from build123d import *

# Parameters (mm, degrees)
SKETCH1_4_R         = 20
SKETCH1_4_R_2       = 15
SKETCH1_4_R_3       = 40
SKETCH1_4_R_4       = 32
SKETCH1_4_R_5       = 21
SKETCH1_4_R_6       = 16
BOSS_EXTRUDE2_DEPTH = 17.5
SKETCH1_5_R         = 15
BOSS_EXTRUDE3_DEPTH = 7.5


with BuildPart() as part:
    # Sketch1_4 → Boss-Extrude2 (new, symmetric)
    # profile 1 of 10: a face of its own
    with BuildSketch(Plane.XY):
        with Locations((-70, 0)):
            Circle(SKETCH1_4_R)
        with Locations((-70, 0)):
            Circle(SKETCH1_4_R_2, mode=Mode.SUBTRACT)
    # profile 2 of 10: a face of its own
    with BuildSketch(Plane.XY):
        with Locations((70, 0)):
            Circle(SKETCH1_4_R)
        with Locations((70, 0)):
            Circle(SKETCH1_4_R_2, mode=Mode.SUBTRACT)
    # profile 3 of 10: a face of its own
    with BuildSketch(Plane.XY):
        Circle(SKETCH1_4_R_3)
        Circle(SKETCH1_4_R_4, mode=Mode.SUBTRACT)
    # profile 4 of 10: a face of its own
    with BuildSketch(Plane.XY):
        with BuildLine():
            ThreePointArc((3, 31.859064644), (0, 32), (-3, 31.859064644))
            Line((-3, 31.859064644), (-3, 20.784609691))
            ThreePointArc((-3, 20.784609691), (0, 21), (3, 20.784609691))
            Line((3, 20.784609691), (3, 31.859064644))
        make_face()
    # profile 5 of 10: a face of its own
    with BuildSketch(Plane.XY):
        with BuildLine():
            ThreePointArc((29.090759323, 13.331456111), (27.712812921, 16), (26.090759323, 18.527608533))
            Line((26.090759323, 18.527608533), (16.5, 12.990381057))
            ThreePointArc((16.5, 12.990381057), (18.186533479, 10.5), (19.5, 7.794228634))
            Line((19.5, 7.794228634), (29.090759323, 13.331456111))
        make_face()
    # profile 6 of 10: a face of its own
    with BuildSketch(Plane.XY):
        with BuildLine():
            Line((16.5, -12.990381057), (26.090759323, -18.527608533))
            ThreePointArc((26.090759323, -18.527608533), (27.712812921, -16), (29.090759323, -13.331456111))
            Line((29.090759323, -13.331456111), (19.5, -7.794228634))
            ThreePointArc((19.5, -7.794228634), (18.186533479, -10.5), (16.5, -12.990381057))
        make_face()
    # profile 7 of 10: a face of its own
    with BuildSketch(Plane.XY):
        with BuildLine():
            Line((-3, -20.784609691), (-3, -31.859064644))
            ThreePointArc((-3, -31.859064644), (0, -32), (3, -31.859064644))
            Line((3, -31.859064644), (3, -20.784609691))
            ThreePointArc((3, -20.784609691), (0, -21), (-3, -20.784609691))
        make_face()
    # profile 8 of 10: a face of its own
    with BuildSketch(Plane.XY):
        with BuildLine():
            Line((-19.5, -7.794228634), (-29.090759323, -13.331456111))
            ThreePointArc((-29.090759323, -13.331456111), (-27.712812921, -16), (-26.090759323, -18.527608533))
            Line((-26.090759323, -18.527608533), (-16.5, -12.990381057))
            ThreePointArc((-16.5, -12.990381057), (-18.186533479, -10.5), (-19.5, -7.794228634))
        make_face()
    # profile 9 of 10: a face of its own
    with BuildSketch(Plane.XY):
        with BuildLine():
            ThreePointArc((-26.090759323, 18.527608533), (-27.712812921, 16), (-29.090759323, 13.331456111))
            Line((-29.090759323, 13.331456111), (-19.5, 7.794228634))
            ThreePointArc((-19.5, 7.794228634), (-18.186533479, 10.5), (-16.5, 12.990381057))
            Line((-16.5, 12.990381057), (-26.090759323, 18.527608533))
        make_face()
    # profile 10 of 10: a face of its own
    with BuildSketch(Plane.XY):
        Circle(SKETCH1_4_R_5)
        Circle(SKETCH1_4_R_6, mode=Mode.SUBTRACT)
    extrude(amount=BOSS_EXTRUDE2_DEPTH, both=True)

    # Sketch1_5 → Boss-Extrude3 (add, symmetric)
    # profile 1 of 2: a face of its own
    with BuildSketch(Plane.XY):
        with BuildLine():
            ThreePointArc((-29.089532552, -61.937098635), (-20.55564481, -45.574895377), (-3, -39.88734135))
            ThreePointArc((-3, -39.88734135), (-40, 0), (-3, 39.88734135))
            ThreePointArc((-3, 39.88734135), (-20.55564481, 45.574895377), (-29.089532552, 61.937098635))
            ThreePointArc((-29.089532552, 61.937098635), (-47.761832891, 80.880388119), (-70.02485881, 66.324952937))
            Line((-70.02485881, 66.324952937), (-89.071294105, 6.023764702))
            ThreePointArc((-89.071294105, 6.023764702), (-66.95253237, 19.766460003), (-50, 0))
            ThreePointArc((-50, 0), (-66.95253237, -19.766460003), (-89.071294105, -6.023764702))
            Line((-89.071294105, -6.023764702), (-70.02485881, -66.324952937))
            ThreePointArc((-70.02485881, -66.324952937), (-47.761832891, -80.880388119), (-29.089532552, -61.937098635))
        make_face()
        with Locations((-50, -60)):
            Circle(SKETCH1_5_R, mode=Mode.SUBTRACT)
        with Locations((-50, 60)):
            Circle(SKETCH1_5_R, mode=Mode.SUBTRACT)
    # profile 2 of 2: a face of its own
    with BuildSketch(Plane.XY):
        with BuildLine():
            Line((70.02485881, -66.324952937), (89.071294105, -6.023764702))
            ThreePointArc((89.071294105, -6.023764702), (50, 0), (89.071294105, 6.023764702))
            Line((89.071294105, 6.023764702), (70.02485881, 66.324952937))
            ThreePointArc((70.02485881, 66.324952937), (47.761832891, 80.880388119), (29.089532552, 61.937098635))
            ThreePointArc((29.089532552, 61.937098635), (20.55564481, 45.574895377), (3, 39.88734135))
            ThreePointArc((3, 39.88734135), (29.325756597, 27.202941017), (40, 0))
            ThreePointArc((40, 0), (29.325756597, -27.202941017), (3, -39.88734135))
            ThreePointArc((3, -39.88734135), (20.55564481, -45.574895377), (29.089532552, -61.937098635))
            ThreePointArc((29.089532552, -61.937098635), (47.761832891, -80.880388119), (70.02485881, -66.324952937))
        make_face()
        with Locations((50, -60)):
            Circle(SKETCH1_5_R, mode=Mode.SUBTRACT)
        with Locations((50, 60)):
            Circle(SKETCH1_5_R, mode=Mode.SUBTRACT)
    extrude(amount=BOSS_EXTRUDE3_DEPTH, both=True)


solid = part.part
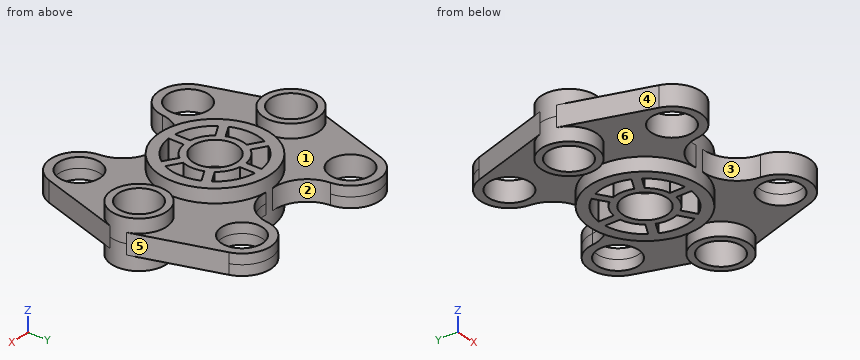
Geometry check sheet. Reference: the model listing, model coordinates, mm. Face numbers are marked on the shaded views. A direction names the side the tool comes from. Give positions to 0.01 mm unless a question says otherwise; leave off trailing zeros. Write each loop counter-clockwise with the first axis right and the second up, starting at its lowest first coordinate (ties: lowest second). Pieces come first, ordered by that corner, then holes.
1) Cross-section at D-D (x = -46). Record the boundary of the cut face in (y, z).
Values follow:
outline: (-80.62, -7.5) - (-74.46, -7.5) - (-74.46, 7.5) - (-80.62, 7.5) - close; (-45.54, -7.5) - (45.54, -7.5) - (45.54, 7.5) - (-45.54, 7.5) - close; (74.46, -7.5) - (80.62, -7.5) - (80.62, 7.5) - (74.46, 7.5) - close
2) Thickness scan on line 1 (Y direction, x = -54.5, z = -2); line 2 (Y direction, x = 39, z = 6.5); line 3 (Y direction, x = -14, z = 13). Record the ranges inside material, lowest first.
Values follow:
line 1: y = -80.51 to -74.31, -45.69 to 45.69, 74.31 to 80.51
line 2: y = -77.89 to -70.2, -49.8 to 49.8, 70.2 to 77.89
line 3: y = -37.47 to -28.77, -15.65 to -7.75, 7.75 to 15.65, 28.77 to 37.47
3) Cross-section at A-A (z = -12.5). Count the separate pieces of the cut face and the enclosed holes in it, plus the area to 3 significant figures.
Values follow:
separate pieces: 3
enclosed holes: 9
area: 3,890 mm2
4) Go/stop test with flat-tipped pins: pin 1 Ø18 at (x, y) = (-50, -60) entering from -Z; pin 2 Ø5.5 at (y, z) = (-27, -7.5) entering from -X; pin 3 Ø9 at (y, z) = (28.5, -5.5) entering from +X; pin 4 Ø5.5 at (y, z) = (24.5, -7) entering from -X. Record where each tip stops, or that it passes through.
Values follow:
pin 1: passes through
pin 2: stops at x = -83.31
pin 3: stops at x = 83.39
pin 4: stops at x = -84.1
5) Release check for a two-part mould opening along X. For the marked faces 4, 5 and 6 record: released by +X, released by -X, zero draft, split by the parting line, or undercut.
Values follow:
face 4: released by -X
face 5: released by +X
face 6: undercut
6) Cross-section at B-B (x = 0). Record the boundary of the cut face in (y, z).
Values follow:
outline: (-40, -17.5) - (-16, -17.5) - (-16, 17.5) - (-40, 17.5) - close; (16, -17.5) - (40, -17.5) - (40, 17.5) - (16, 17.5) - close
7) Set-up check for the marked faces 1, 2 and 3: record each of +Z, -Z, +X, -X, +Y, -Y from which the full face is reachable in a straight line by a thin tool's end or side.
Values follow:
face 1: +Z
face 2: +Z, -Z, +Y
face 3: +Z, -Z, -Y
8) Cross-section at C-C (y = 54.5). Record the boundary of the cut face in (x, z).
Values follow:
outline: (-73.76, -7.5) - (-63.96, -7.5) - (-63.96, 7.5) - (-73.76, 7.5) - close; (-36.04, -7.5) - (-27.19, -7.5) - (-27.19, 7.5) - (-36.04, 7.5) - close; (27.19, -7.5) - (36.04, -7.5) - (36.04, 7.5) - (27.19, 7.5) - close; (63.96, -7.5) - (73.76, -7.5) - (73.76, 7.5) - (63.96, 7.5) - close
